Autodesk Inventor part; units mm, degrees
ref_plane "YZ Plane" through (0, 0, 0) normal (1, 0, 0) x (0, 1, 0)
ref_plane "XZ Plane" through (0, 0, 0) normal (0, 1, 0) x (-1, 0, 0)
ref_plane "XY Plane" through (0, 0, 0) normal (0, 0, 1) x (1, 0, 0)
sketch "Sketch2" plane through (0, 0, 0) normal (1, 0, 0) x (0, 1, 0)
  line L0 (0, 0) -> (14, 0)
  line L1 (14, 0) -> (16.5, 0)
  line L2 (14, 0) -> (11.5, 0)
  line L3 (14, 0) -> (28, 0)
  line L4 (14, 0) -> (-8.55, 0)
  circle A0 centre (14, 0) radius 2.75
  line L5 (-8.55, 0) -> (-8.55, 8.8)
  line L6 (-8.55, 0) -> (-8.55, -8.8)
  line L7 (0, 0) -> (0, -13.3)
  line L8 (0, -13.3) -> (6.5, -13.3)
  line L9 (0, 0) -> (0, 13.3)
  line L10 (28, 0) -> (29.5, 0)
  line L11 (29.5, 0) -> (32.5, 0)
  line L12 (-10.05, 10.3) -> (-13.05, 10.3)
  line L13 (-13.05, 10.3) -> (-13.05, 13.3)
  line L14 (-13.05, 13.3) -> (-10.05, 13.3)
  line L15 (-10.05, 13.3) -> (-10.05, 10.3)
  line L16 (-10.05, -10.3) -> (-13.05, -10.3)
  line L17 (-13.05, -10.3) -> (-13.05, -13.3)
  line L18 (-13.05, -13.3) -> (-10.05, -13.3)
  line L19 (-10.05, -13.3) -> (-10.05, -10.3)
  line L20 (-13.05, -13.3) -> (32.5, -13.3)
  line L21 (32.5, -13.3) -> (32.5, 13.3)
  line L22 (32.5, 13.3) -> (-13.05, 13.3)
  line L23 (-13.05, 13.3) -> (-13.05, -13.3)
  line L24 (9.5, 13.3) -> (-3, 13.3)
  circle A1 centre (14, 0) radius 7.5
  line L25 (28, 0) -> (25.6, 0)
  line L26 (25.6, 0) -> (25.6, -2.4)
  line L27 (25.6, 2.4) -> (25.6, -2.4)
  line L28 (25.6, 13.3) -> (25.6, -13.3)
  line L29 (32.5, 0) -> (32.5, -3)
  line L30 (28, -1.5) -> (28, -4.5)
  line L31 (28, 1.5) -> (28, 4.5)
  line L32 (32.5, 4.5) -> (25.6, 4.5)
  line L33 (25.6, 4.5) -> (25.6, -4.5)
  line L34 (25.6, -4.5) -> (32.5, -4.5)
  line L35 (32.5, -4.5) -> (32.5, 4.5)
  line L36 (0, -13.3) -> (0, -38.3)
  line L37 (0, -38.3) -> (6.5, -38.3)
  line L38 (6.5, -13.3) -> (9.5, -13.3)
  line L39 (9.5, -13.3) -> (9.5, -38.3)
  line L40 (9.5, -38.3) -> (6.5, -38.3)
  line L41 (6.5, -38.3) -> (6.5, -13.3)
  line L42 (0, -13.3) -> (-3, -13.3)
  line L43 (-3, -13.3) -> (-3, -38.3)
  line L44 (-3, -38.3) -> (0, -38.3)
  line L45 (0, -38.3) -> (0, -13.3)
  line L46 (9.5, -13.3) -> (6.5, -13.3)
  line L47 (6.5, -13.3) -> (6.5, -10.3)
  line L48 (6.5, -10.3) -> (9.5, -10.3)
  line L49 (9.5, -10.3) -> (9.5, -13.3)
  line L50 (-3, -13.3) -> (-3, 13.3)
  line L51 (-7.05, 8.8) -> (-5.05, 8.8)
  line L52 (-4.05, 13.3) -> (-4.05, -13.3)
  line L53 (9.5, -10.3) -> (9.5, 13.3)
  line L54 (6.5, -10.3) -> (6.5, 13.3)
  line L55 (25.6, -7.5) -> (0, -7.5)
  line L56 (25.6, 7.5) -> (0, 7.5)
  line L57 (14, 0) -> (19.3033, -5.3033)
  line L58 (14, 0) -> (21.5, 0) construction
  line L59 (19.3033, -5.3033) -> (14, -10.6066)
  line L60 (14, -10.6066) -> (24.6066, 0)
  line L61 (14, -10.6066) -> (3.3934, 0)
  line L62 (24.6066, 0) -> (14, 10.6066)
  line L63 (14, 10.6066) -> (3.3934, 0)
  line L64 (0, 13.3) -> (-1, 13.3)
  line L65 (-1, 13.3) -> (-1, -38.3)
  line L66 (-3, -38.3) -> (-4.05, -38.3)
  line L67 (-4.05, -38.3) -> (-4.05, -13.3)
  line L68 (25.6, 0) -> (27.6, 0)
  line L69 (25.6, 0) -> (27.6, 0)
  line L70 (27.6, 0) -> (29.1, 0)
  line L71 (29.1, 0) -> (27.1, 0)
  circle A2 centre (28, 0) radius 1.5
  circle A3 centre (-7.05, 8.8) radius 1.5
  circle A4 centre (-7.05, -8.8) radius 1.5
  point P0 (-3, -13.3)
  point P1 (6.5, 10.3)
  point P2 (6.5, -7.5)
  point P3 (6.5, 7.5)
  point P4 (6.5, -3.1066)
  point P5 (10.8934, -7.5)
  point P6 (6.5, 3.1066)
  point P7 (10.8934, 7.5)
  point P8 (17.1066, -7.5)
  point P9 (17.1066, 7.5)
  dimension "d30" = 15
  dimension "d8" = 14
  dimension "d9" = 2.5
  dimension "d10" = 2.5
  dimension "d11" = 14
  dimension "d12" = 22.55
  dimension "d14" = 5.5
  dimension "d15" = 8.8
  dimension "d19" = 13.3
  dimension "d23" = 3
  dimension "d24" = 3
  dimension "d25" = 3
  dimension "d26" = 3
  dimension "d27" = 3
  dimension "d39" = 3
  dimension "d42" = 25
  dimension "d43" = 6.5
  dimension "d44" = 3
  dimension "d45" = 3
  dimension "d46" = 3
  dimension "d47" = 2
  dimension "d55" = 45
  dimension "d58" = 15
  dimension "d64" = 1
  dimension "d65" = 2
  dimension "d66" = 1.5
  dimension "d68" = 2
  dimension "d70" = 3
  dimension "d71" = 3
extrude "Extrusion1" add sketch "Sketch2" along normal blind 8.6 contours L65 L20 L50 L4 | L4 L50 L22 L65 | L50 L20 L52 L4 | L4 L52 L22 L50 | L65 L44 L43 L20 | L43 L66 L67 L20 | L47 L48 L49 L20 | L20 L39 L40 L41
extrude "Extrusion2" add sketch "Sketch2" against normal blind 9.5 contours L9 L56 L54 L63 L0 | L7 L20 L65 L4 | L0 L61 L54 L55 L7 | L4 L65 L22 L9 | L65 L20 L50 L4 | L4 L50 L22 L65 | L55 L54 L47 L8 L7 | L9 L22 L54 L56 | L61 L53 L55 L54 | L54 L56 L53 L63 | L50 L20 L52 L4 | L4 L52 L22 L50 | L55 L53 L48 L54 | L54 L22 L53 L56 | L47 L48 L49 L20 | L55 L61 L59 L28 L20 L49 L53 | L53 L61 L55 | L56 L63 L53 | L53 L22 L28 L56 L62 L63 | L60 L3 L26 L28 L55 L59 | L62 L56 L28 L27 L3
extrude "Extrusion3" add sketch "Sketch2" along normal blind 3 from surface at -9.5 contours L52 L20 L19 L16 L23 L12 L15 L22 | L15 L12 L13 L14 | L18 L17 L16 L19 | L28 L34 L21 L20 | L22 L21 L32 L28 | L34 L30 A2 L11 L21 | L28 L26 L3 A2 L30 L34 | L21 L11 A2 L31 L32 | L32 L31 A2 L3 L27 L28
extrude "Extrusion4" add sketch "Sketch2" along normal blind 3 from surface at 8.6 contours L9 L56 L54 L63 L0 | L7 L20 L65 L4 | L0 L61 L54 L55 L7 | L4 L65 L22 L9 | L63 L54 L0 | L0 L54 L61 | L65 L20 L50 L4 | L4 L50 L22 L65 | L55 L54 L47 L8 L7 | L9 L22 L54 L56 | A1 L53 L0 | L54 L63 A1 | L0 L53 A1 | A1 L61 L54 | L61 L53 L55 L54 | L54 L56 L53 L63 | L50 L20 L52 L4 | L4 L52 L22 L50 | L65 L44 L43 L20 | L20 L36 L44 L65 | L8 L41 L37 L36 | L55 L53 L48 L54 | L54 L22 L53 L56 | L63 L53 A1 | A1 L53 L61 | L43 L66 L67 L20 | L47 L48 L49 L20 | L20 L39 L40 L41
sketch "Sketch3" plane through (0, 9.5, -13.3) normal (0, 1, 0) x (1, 0, 0)
  line L0 (0, -3) -> (8.6, -3)
  line L1 (8.6, -3) -> (0, 5.6)
  line L2 (0, 25) -> (0, 0)
  line L3 (8.6, -3) -> (20.7622, -3) construction
  line L4 (0, 5.6) -> (0, -3)
  line L5 (0, 0) -> (0, -26.6)
  line L6 (8.6, -3) -> (0, -3)
  point P0 (0, -13.3)
  point P1 (0, 0)
  dimension "d59" = 135
extrude "Extrusion5" cut sketch "Sketch3" against normal up to next
extrude "Extrusion6" add sketch "Sketch2" against normal blind 3 contours L65 L44 L43 L20 | L20 L36 L44 L65 | L8 L41 L37 L36 | L43 L66 L67 L20 | L20 L39 L40 L41
properties part number "linear motion motor and gearbox holder"
Could you check a few things on this model? Use its own coordinates, in mm. A direction names the side the tool comes from. Give positions to 0.01 mm unless a question says otherwise; leave off trailing zeros. Order: outer loops, then holes, each group sorted by start corner. A loop starts at its lowest first (then second) coordinate and runs counter-clockwise, first axis right, second up. Notation, with made-up numbers: (46.25, 47.5) - (67.25, 47.5) arc R24 cw to (67.25, 72.5) - close; hole circle Ø10 at (33.25, 60). An arc over 180 degrees is marked (long way). One line per question, with ' | ' between items. Start each with the question number.
Item 1: Thinking about a two-plate mould opening in Y: for faces 4 (the flat face through (-4.684, 19.378, 5.229)), 5 (the flat face through (-9.5, 4, 3)), 6 (the flat face through (6, 9.5, -19)), which applies, pulls with the +Y half, pulls with the -Y half, needs draft (parallel to the pull), parting line crosses it, or undercut?
Item 2: I need wall thicknesses on probe 1 along Y at (x, z) = (5, -30.5); probe 2 along X at (y, z) = (0, -11.5); probe 3 along Y at (x, z) = (-7.35, 8.8). Which ranges of each line are inside material? Lowest first, please. Write a range as [from, to].
Item 3: For faces 1 (the flat face through (4, 6.5, -28)), 2 (the flat face through (8.6, 3, -12)), 3 (the flat face through (-4.684, 8.771, 5.378)), which set-ups out of +Z, -Z, +X, -X, +Y, -Y let a thin tool reach every point of the face, with its end or its side?
Item 4: I want a section at B-B on y = -7.05. Write out the boundary of the cut face in (x, z), then the cut area to 3 significant figures.
Item 5: I want a section at C-C on z = -8.8. Write out the boundary of the cut face in (x, y), then the cut area to 3 significant figures.
Item 6: I want a section at D-D on x = -3.75. Write out the boundary of the cut face in (y, z), then the cut area to 3 significant figures.
Item 7: I'm going to push flat-ended pins straight in: pin 1 Ø4 at (y, z) = (28, 0) entering from +X; pin 2 Ø2 at (x, z) = (-4.5, 2) entering from +Y; pin 3 Ø2 at (y, z) = (11.5, -5.5) entering from -X; pin 4 Ø1 at (x, z) = (9.5, -26.5) entering from +Y. Where does each tip first touch, or does it pass through?
Item 8: I want a section at A-A on x = 1.25. Write out the boundary of the cut face in (y, z).
Verdict:
1) face 4: undercut | face 5: needs draft | face 6: pulls with the +Y half
2) probe 1: [-4.05, -1], [6.5, 9.5] | probe 2: [-9.5, 0], [8.6, 11.6] | probe 3: [-13.05, -8.55], [-5.55, 12.19], [15.81, 32.5]
3) face 1: +Z, -Z | face 2: +Z | face 3: -X
4) outline: (-9.5, -13.3) - (-6.5, -13.3) - (-6.5, -10.3) - (-9.5, -10.3) - close; (-9.5, -7.3) - (-6.5, -7.3) - (-6.5, 7.3) - (-9.5, 7.3) - close; (-9.5, 10.3) - (-6.5, 10.3) - (-6.5, 13.3) - (-9.5, 13.3) - close | area: 61.8 mm^2
5) outline: (-9.5, -13.05) - (-6.5, -13.05) - (-6.5, -8.55) - (-9.5, -8.55) - close; (-9.5, -5.55) - (-6.5, -5.55) - (-6.5, -4.05) - (11.6, -4.05) - (11.6, 9.5) - (8.6, 9.5) - (8.6, -1) - (0, -1) - (0, 12.19) - (-9.5, 12.19) - close; (-9.5, 15.81) - (0, 15.81) - (0, 25.6) - (-6.5, 25.6) - (-6.5, 32.5) - (-9.5, 32.5) - close | area: 353 mm^2
6) outline: (-4.05, -13.3) - (25.6, -13.3) - (25.6, 13.3) - (-4.05, 13.3) - close; hole (3.39, 0) - (14, -10.61) - (24.61, 0) - (14, 10.61) - close | area: 564 mm^2
7) pin 1: x = -6.5 | pin 2: y = 25.6 | pin 3: through | pin 4: y = 9.5
8) outline: (-4.05, -38.3) - (-1, -38.3) - (-1, 13.3) - (-4.05, 13.3) - close; (6.5, -38.3) - (9.5, -38.3) - (9.5, -17.65) - (6.5, -17.65) - close
